The listing builds one solid part. Answer for the finished solid, in the listing's coordinates (mm). Face numbers are marked on the shaded views. A direction names the side the tool comes from. Round coordinates to 2 decimals unless told otherwise and drop trailing zeros. Loops run counter-clockwise (first coordinate to the right, second up) from the corner with the lowest first, then second, coordinate; pieces in that order, holes last. Notation, with made-up numbers: (-36, 72.25) -> (-23, 72.25) arc R23 cw to (-23, 80.25) -> close; hole circle Ø6 at (81.25, 52). An arc over 180 degrees is marked (long way). Answer in a Markdown table with one row per item. Add a question column.
```python
from build123d import *

# Parameters (mm, degrees)
BOSS_EXTRUDE1_DEPTH = 5
BOSS_EXTRUDE2_START = -5
SKETCH2_3_W         = 1.5
SKETCH2_3_H         = 1.5
BOSS_EXTRUDE2_DEPTH = 5
FILLET1_R           = 1
CUT_EXTRUDE1_START  = -5
SKETCH3_R           = 1.35
CUT_EXTRUDE1_DEPTH  = 4


with BuildPart() as part:
    # Sketch2 → Boss-Extrude1 (new body)
    with BuildSketch(Plane(origin=(0, 0, 0), x_dir=(1, 0, 0), z_dir=(0, 1, 0))):
        with BuildLine():
            ThreePointArc((-8, 1.5), (-7.267766953, 3.267766953), (-5.5, 4))
            Line((-5.5, 4), (5.5, 4))
            ThreePointArc((5.5, 4), (7.267766953, 3.267766953), (8, 1.5))
            Line((8, 1.5), (8, -1.5))
            ThreePointArc((8, -1.5), (7.267766953, -3.267766953), (5.5, -4))
            Line((5.5, -4), (-5.5, -4))
            ThreePointArc((-5.5, -4), (-7.267766953, -3.267766953), (-8, -1.5))
            Line((-8, -1.5), (-8, 1.5))
        make_face()
    extrude(amount=BOSS_EXTRUDE1_DEPTH)

    # Sketch2<3> → Boss-Extrude2 (add)
    # profile 1 of 4: a face of its own
    with BuildSketch(Plane(origin=(0, 0, 0), x_dir=(1, 0, 0), z_dir=(0, 1, 0)).offset(BOSS_EXTRUDE2_START)):
        Polygon((-10, 6.5), (-10, 0.75), (-10, -0.75), (-10, -6.5), (10, -6.5), (10, -0.75), (10, 0.75), (10, 6.5), align=None)
        with BuildLine():
            ThreePointArc((-8, 1.5), (-7.267766953, 3.267766953), (-5.5, 4))
            Line((-5.5, 4), (5.5, 4))
            ThreePointArc((5.5, 4), (7.267766953, 3.267766953), (8, 1.5))
            Line((8, 1.5), (8, -1.5))
            ThreePointArc((8, -1.5), (7.267766953, -3.267766953), (5.5, -4))
            Line((5.5, -4), (-5.5, -4))
            ThreePointArc((-5.5, -4), (-7.267766953, -3.267766953), (-8, -1.5))
            Line((-8, -1.5), (-8, 1.5))
        make_face(mode=Mode.SUBTRACT)
    # profile 2 of 4: a face of its own
    with BuildSketch(Plane(origin=(0, 0, 0), x_dir=(1, 0, 0), z_dir=(0, 1, 0)).offset(BOSS_EXTRUDE2_START)):
        with BuildLine():
            ThreePointArc((-8, 1.5), (-7.267766953, 3.267766953), (-5.5, 4))
            Line((-5.5, 4), (5.5, 4))
            ThreePointArc((5.5, 4), (7.267766953, 3.267766953), (8, 1.5))
            Line((8, 1.5), (8, -1.5))
            ThreePointArc((8, -1.5), (7.267766953, -3.267766953), (5.5, -4))
            Line((5.5, -4), (-5.5, -4))
            ThreePointArc((-5.5, -4), (-7.267766953, -3.267766953), (-8, -1.5))
            Line((-8, -1.5), (-8, 1.5))
        make_face()
    # profile 3 of 4: a face of its own
    with BuildSketch(Plane(origin=(0, 0, 0), x_dir=(1, 0, 0), z_dir=(0, 1, 0)).offset(BOSS_EXTRUDE2_START)):
        with Locations((10.75, 0)):
            Rectangle(SKETCH2_3_W, SKETCH2_3_H)
    # profile 4 of 4: a face of its own
    with BuildSketch(Plane(origin=(0, 0, 0), x_dir=(1, 0, 0), z_dir=(0, 1, 0)).offset(BOSS_EXTRUDE2_START)):
        with Locations((-10.75, 0)):
            Rectangle(SKETCH2_3_W, SKETCH2_3_H)
    extrude(amount=BOSS_EXTRUDE2_DEPTH)

    # Fillet1
    fillet1_edges = [part.edges().sort_by_distance(p)[0] for p in [
        (-8, 5, 0),
        (-7.267766953, 5, 3.267766953),
        (0, 5, 4),
        (7.267766953, 5, 3.267766953),
        (8, 5, 0),
        (7.267766953, 5, -3.267766953),
        (0, 5, -4),
        (-7.267766953, 5, -3.267766953),
    ]]
    fillet(fillet1_edges, radius=FILLET1_R)

    # Sketch3 → Cut-Extrude1 (cut)
    with BuildSketch(Plane(origin=(0, 0, 0), x_dir=(1, 0, 0), z_dir=(0, 1, 0)).offset(CUT_EXTRUDE1_START)):
        with Locations((10, 0)):
            Circle(SKETCH3_R)
        with Locations((-10, 0)):
            Circle(SKETCH3_R)
    extrude(amount=CUT_EXTRUDE1_DEPTH, mode=Mode.SUBTRACT)


solid = part.part
```
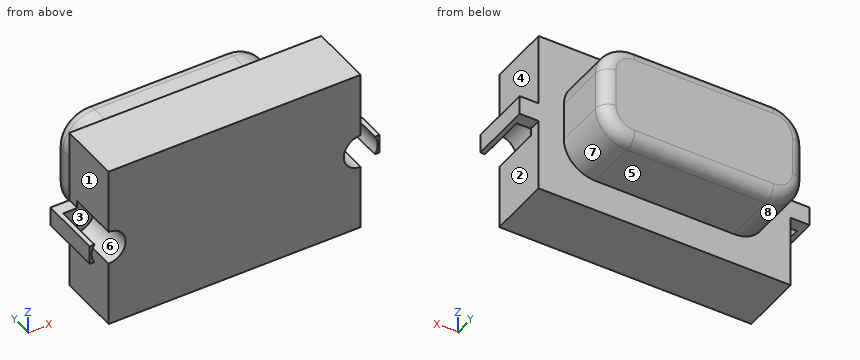
Item 1: Consider L1, parallel to X at y = -0.25, z = -3; L2, parallel to Z at x = -5, y = 1; L3, parallel to Y at x = 5, z = 6. Determine where each line is inside the solid, lowest interval first. Write a range as from..to.
Item 2: Flat-ended cylindrical pins translate along their axes: P1, Ø2.5, axis at y = -2.5, z = 3.5, coming from the -X side; P2, Ø1.6, axis at x = 11, y = -3, coming from the -Z side; P3, Ø5.5, axis at y = -2.5, z = 5, coming from the +X side. Find the tip coordinate at first contact, or state that the pin passes through.
Item 3: Section C-C, the plane x = -0.5 is taken. Write down the section's boundary in (y, z), and give its area (3 significant figures).
Item 4: Section D-D, the plane y = 1.25 is taken. Write down the section's boundary in (x, z), and give its area (3 significant figures).
Item 5: The mould has two halves that part along X. Classify the marked faces 6, 7 and 8: +X half, -X half, draft (parallel to the pull), parting line (faces both ways), or undercut.
Item 6: Section A-A, the plane y = -2 is taken. Write down the section's boundary in (x, z), and give its area (3 significant figures).
Item 7: For the marked faces 1, 2, 3, 4 and 5, determine the directions among +Z, -Z, +X, -X, +Y, -Y from which every point of the face is accessible in a straight line to the end or side of a thin tool.
Item 8: Section B-B, the plane z = 0 is taken. Write down the section's boundary in (x, y).
Here are the results:
| question | item | result |
|---|---|---|
| 1 | L1 | x = -10..10 |
| 1 | L2 | z = -4..4 |
| 1 | L3 | y = -5..0 |
| 2 | P1 | stops at x = -10 |
| 2 | P2 | stops at z = -0.75 |
| 2 | P3 | stops at x = 10 |
| 3 | outline | (-5, -6.5) -> (0, -6.5) -> (0, -4) -> (4, -4) arc R1 ccw to (5, -3) -> (5, 3) arc R1 ccw to (4, 4) -> (0, 4) -> (0, 6.5) -> (-5, 6.5) -> close |
| 3 | area | 105 mm² |
| 4 | outline | (-8, -1.5) arc R2.5 ccw to (-5.5, -4) -> (5.5, -4) arc R2.5 ccw to (8, -1.5) -> (8, 1.5) arc R2.5 ccw to (5.5, 4) -> (-5.5, 4) arc R2.5 ccw to (-8, 1.5) -> close |
| 4 | area | 123 mm² |
| 5 | face 6 | undercut |
| 5 | face 7 | +X half |
| 5 | face 8 | -X half |
| 6 | outline | (-11.5, -0.75) -> (-11.12, -0.75) arc R1.35 cw to (-11.12, 0.75) -> (-11.5, 0.75) -> close; (-10, -6.5) -> (10, -6.5) -> (10, -1.35) arc R1.35 cw to (10, 1.35) -> (10, 6.5) -> (-10, 6.5) -> (-10, 1.35) arc R1.35 cw to (-10, -1.35) -> close; (11.12, -0.75) -> (11.5, -0.75) -> (11.5, 0.75) -> (11.12, 0.75) arc R1.35 cw to start |
| 6 | area | 255 mm² |
| 7 | face 1 | +Z, -X, +Y, -Y |
| 7 | face 2 | -Z, +X, +Y, -Y |
| 7 | face 3 | -Y |
| 7 | face 4 | +Z, +X, +Y, -Y |
| 7 | face 5 | -Z, +X, -X, +Y |
| 8 | outline | (-11.5, -5) -> (-11.35, -5) -> (-11.35, -1) -> (-8.65, -1) -> (-8.65, -5) -> (8.65, -5) -> (8.65, -1) -> (11.35, -1) -> (11.35, -5) -> (11.5, -5) -> (11.5, 0) -> (8, 0) -> (8, 4) arc R1 ccw to (7, 5) -> (-7, 5) arc R1 ccw to (-8, 4) -> (-8, 0) -> (-11.5, 0) -> close |
